Design review of the part built by this model. Coordinates are the model's own, in mm. Face numbers are marked on the shaded views. Coordinates: 2 decimals unless noted, no trailing zeros. Loops run counter-clockwise (first coordinate to the right, second up) from the corner with the lowest first, then second, coordinate; pieces in that order, holes last. Notation, with made-up numbers: (88.25, 10) -> (140.25, 10) arc R20 ccw to (140.25, 25) -> close; hole circle Ø3 at (45, -36.5). An arc over 180 degrees is marked (long way). Use CSV: the item, a comma, the result in double quotes.
```python
from build123d import *

# Parameters (mm, degrees)
F0_W       = 800
F0_H       = 400
F1_DEPTH   = 400
F2_W       = 300
F2_H       = 350
F3_DEPTH   = 800.001
F4_W       = 700
F4_H       = 350
F5_DEPTH   = 400.001
F8_W       = 800
F8_H       = 300
F9_DEPTH   = 50
F10_W      = 700
F10_H      = 300
F11_DEPTH  = 446.7348071841
F12_DEPTH  = 8.8163490354
F11_FACE_W = 50
F11_FACE_H = 50
F15_DEPTH  = 200


with BuildPart() as f1:
    # F0 (on Top) → F1 (new body)
    with BuildSketch(Plane.XY):
        Rectangle(F0_W, F0_H)
    extrude(amount=F1_DEPTH)

    # F2 (on face) → F3 (cut, through all)
    with BuildSketch(Plane.YZ.offset(400)):
        with Locations((0, 175)):
            Rectangle(F2_W, F2_H)
    extrude(amount=-F3_DEPTH, mode=Mode.SUBTRACT)

    # F4 (on face) → F5 (cut, through all)
    with BuildSketch(Plane.XZ.offset(200)):
        with Locations((0, 175)):
            Rectangle(F4_W, F4_H)
    extrude(amount=-F5_DEPTH, mode=Mode.SUBTRACT)



with BuildPart() as f9:
    # F8 (on face) → F9 (new body)
    with BuildSketch(Plane(origin=(0, 125.5652334135, -22.1405384897), x_dir=(1, 0, 0), z_dir=(0, -0.984807753, 0.1736481777))):
        with Locations((0, 578.6527367383)):
            Rectangle(F8_W, F8_H)
    extrude(amount=F9_DEPTH)

    # F10 (on face) → F11 (cut, through all)
    with BuildSketch(Plane(origin=(0, 125.5652334135, -22.1405384897), x_dir=(-1, 0, 0), z_dir=(0, 0.984807753, -0.1736481777))):
        with Locations((0, 578.6527367383)):
            Rectangle(F10_W, F10_H)
    extrude(amount=-F11_DEPTH, mode=Mode.SUBTRACT)


with BuildPart() as f1_1:
    add(f1.part)
    # F12 (add, through all): a face of the model
    f12_faces = [f9.part.faces().sort_by_distance(p)[0] for p in [
        (-375, 175.3798061747, 404.3412044417),
    ]]

    add(f9.part)  # F12 merges F9
    extrude(f12_faces, amount=F12_DEPTH)

    # F11_face (on face) → F13 (join, up to the next surface of F1)
    with BuildSketch(Plane(origin=(-375, 175.3798061747, 404.3412044417), x_dir=(1, 0, 0), z_dir=(0, -0.1736481777, -0.984807753))):
        with Locations((750, 0)):
            Rectangle(F11_FACE_W, F11_FACE_H)
    extrude(until=Until.NEXT)

    # F14 (on face) → F15 (join)
    with BuildSketch(Plane(origin=(0, 126.5292198866, 717.5828643934), x_dir=(1, 0, 0), z_dir=(0, 0.1736481777, 0.984807753))):
        with BuildLine():
            ThreePointArc((-350, 77.5022795357), (0, 190.1625622952), (350, 77.5022795357))
            Line((350, 77.5022795357), (350, 107.9704417254))
            ThreePointArc((350, 107.9704417254), (-8.8874458979, 215.0993697449), (-364.5833333333, 97.8081010874))
            Line((-364.5833333333, 97.8081010874), (-350, 77.5022795357))
        make_face()
    extrude(amount=-F15_DEPTH)


solid = f1_1.part
```
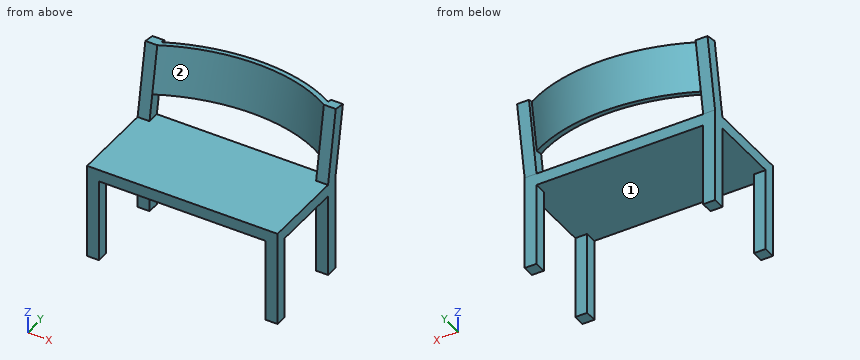
Item 1: Add section B-B (y = -161). Give the boundary of the cut face in (x, z), then the cut area to 3 significant figures.
Checked values:
outline,"(-400, 0) -> (-350, 0) -> (-350, 350) -> (350, 350) -> (350, 0) -> (400, 0) -> (400, 400) -> (-400, 400) -> close"
area,"75,000 mm^2"
Item 2: Add section C-C (x = -259). Give the boundary of the cut face in (y, z).
Checked values:
outline,"(-200, 350) -> (200, 350) -> (200, 400) -> (-200, 400) -> close; (221.19, 497.81) -> (248.36, 493.02) -> (283.09, 689.98) -> (255.92, 694.77) -> close"
Item 3: Add section D-D (z = 452.5). Give the boundary of the cut face in (x, y), then the cut area to 3 significant figures.
Checked values:
outline,"(-400, 158.49) -> (-350, 158.49) -> (-350, 209.26) -> (-400, 209.26) -> close; (350, 158.49) -> (400, 158.49) -> (400, 209.26) -> (350, 209.26) -> close"
area,"5,080 mm^2"
Item 4: Clearance check with flat-ended pins moving along their axes: pin 1 (2 mm diameter, centred on x = -170, y = 190, fed in from +Z); pin 2 (12 mm diameter, centred on x = 264.5, z = 577, fed in from -Y); pin 3 (15 mm diameter, centred on x = -375, z = 130, fed in from +Y). State where each tip first meets the part, or that it passes through.
Checked values:
pin 1,"z = 400"
pin 2,"y = 229.23"
pin 3,"y = 200"
Item 5: Add section A-A (z = 142.5). Give the boundary of the cut face in (x, y).
Checked values:
outline,"(-400, -200) -> (-350, -200) -> (-350, -150) -> (-400, -150) -> close; (-400, 150) -> (-350, 150) -> (-350, 200) -> (-400, 200) -> close; (350, -200) -> (400, -200) -> (400, -150) -> (350, -150) -> close; (350, 150) -> (400, 150) -> (400, 200) -> (350, 200) -> close"
Item 6: To check wall thickness, follow line 1 along Y through (x, z) = (364, 101); line 2 along Z through (x, y) = (48.5, -64.5); line 3 along X through (y, z) = (170.5, 512). State the ranges of each line that lie inside material, in increasing order.
Checked values:
line 1,"-200 to -150, 150 to 200"
line 2,"350 to 400"
line 3,"-400 to -347.9, 347.9 to 400"
Item 7: Draft analysis for pull direction X (two halves, no side actions). For the marked faces 1 and 2, state which applies: pulls with the +X half, pulls with the -X half, needs draft (parallel to the pull), parting line crosses it, or undercut.
Checked values:
face 1,"undercut"
face 2,"undercut"
